The drawing under review shows one solid part. Ordinate dimensions are in mm from its lowest x, y, z. A direction names the side the tool comes from. Coordinates: 2 decimals unless noted, no trailing zeros. Order: outer loops, then holes, each group sorted by start corner. A loop starts at its lowest first (then second) coordinate and runs counter-clockwise, first axis right, second up. Notation, with made-up numbers: (-5, -36) - (30, -36) arc R6 cw to (30, -27) - close; hole circle Ø1 at (-25, 41.5). An arc over 180 degrees is marked (long way). Answer in a Markdown table with one row per item.
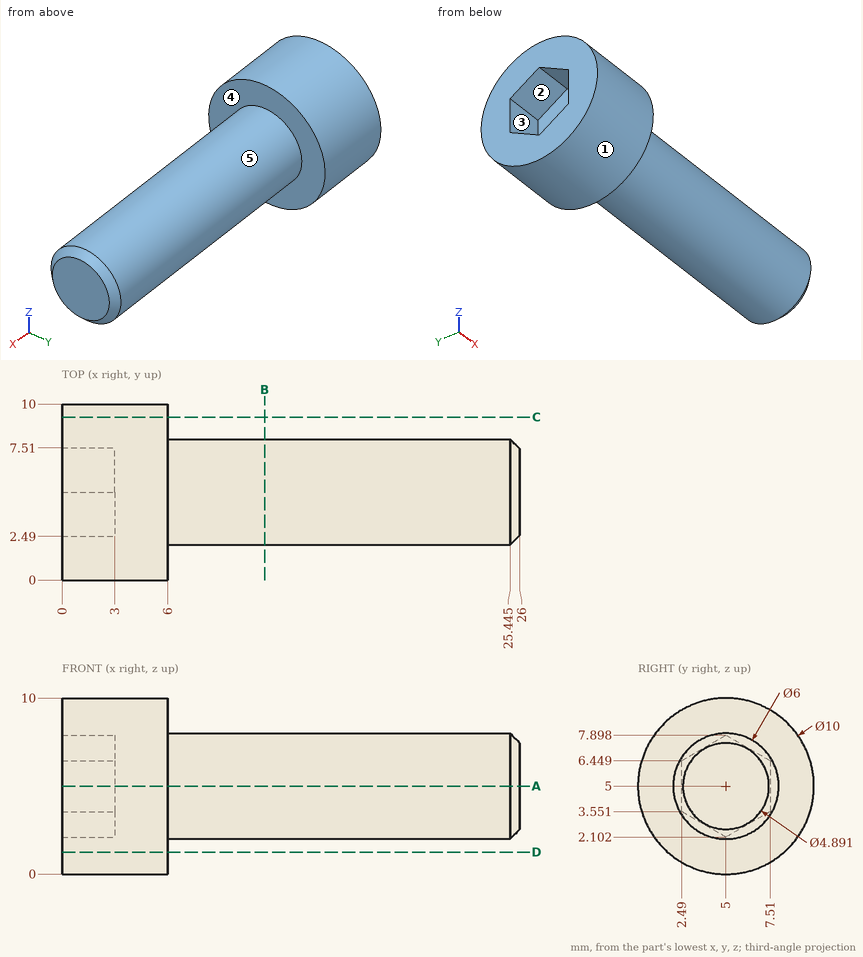
Item 1: We need section C-C, the plane y = 9.25. Write out the cut boundary in (x, z), then the cut area to 3 significant figures.
Check values:
| item | result |
|---|---|
| outline | (0, 2.37) - (6, 2.37) - (6, 7.63) - (0, 7.63) - close |
| area | 31.6 mm^2 |
Item 2: We need section D-D, the plane z = 1.25. Write out the cut boundary in (x, y), then the cut area to 3 significant figures.
Check values:
| item | result |
|---|---|
| outline | (0, 1.69) - (6, 1.69) - (6, 8.31) - (0, 8.31) - close |
| area | 39.7 mm^2 |
Item 3: We need section B-B, the plane x = 11.5. Write out the cut boundary in (y, z), then the cut area to 3 significant figures.
Check values:
| item | result |
|---|---|
| outline | circle Ø6 at (5, 5) |
| area | 28.3 mm^2 |
Item 4: Clearance check with flat-ended pins moving along their axes: pin 1 Ø1.5 at (x, y) = (13, 5.5) entering from +Z; pin 2 Ø3 at (x, z) = (18.5, 3.5) entering from +Y; pin 3 Ø5 at (x, y) = (7, 2.5) entering from +Z; pin 4 Ø2.5 at (y, z) = (5, 3.5) entering from -X. State where each tip first meets the part, or that it passes through.
Check values:
| item | result |
|---|---|
| pin 1 | z = 8 |
| pin 2 | y = 8 |
| pin 3 | z = 10 |
| pin 4 | x = 0 |
Item 5: To check wall thickness, follow line 1 (Y direction, x = 2, z = 2.5); line 2 (Y direction, x = 23, z = 4.25) (1 decimal); line 3 (X direction, y = 5.5, z = 9). State the ranges of each line that lie inside material, in increasing order. Write a range as from..to.
Check values:
| item | result |
|---|---|
| line 1 | 0.67..4.31, 5.69..9.33 |
| line 2 | 2.1..7.9 |
| line 3 | 0..6 |
Item 6: Mouldability with a two-part tool opening along Y and no side actions: class the marked faces 3, 4 and 5 as +Y half, -Y half, draft (parallel to the pull), parting line (faces both ways), or undercut.
Check values:
| item | result |
|---|---|
| face 3 | undercut |
| face 4 | draft |
| face 5 | parting line |
Item 7: Tool access review of the marked faces 1 and 2: name each direction out of +Z, -Z, +X, -X, +Y, -Y from which nothing blocks a thin tool from reaching the whole face with its end or side.
Check values:
| item | result |
|---|---|
| face 1 | +X, -X |
| face 2 | -X |
Item 8: We need section A-A, the plane z = 5. Write out the cut boundary in (x, y) (1 decimal), then the cut area to 3 significant figures.
Check values:
| item | result |
|---|---|
| outline | (0, 0) - (6, 0) - (6, 2) - (25.4, 2) - (26, 2.6) - (26, 7.4) - (25.4, 8) - (6, 8) - (6, 10) - (0, 10) - (0, 7.5) - (3, 7.5) - (3, 2.5) - (0, 2.5) - close |
| area | 165 mm^2 |
